Model file for the job. Use its own axes, mm. Coordinates: 2 decimals unless noted, no trailing zeros. Write each loop counter-clockwise with the first axis right and the second up, starting at its lowest first coordinate (ties: lowest second). Pieces come first, ordered by that corner, then holes. Notation, with made-up numbers: M 66.25,-24.75 L 72.25,-24.75 A21 ccw 72.25,-9.75 Z; hole C -34,83 d10. An arc over 180 degrees is marked long. Put each result on its own line as item: value. Start each with the question number.
Q1. Cut at B-B (x = 92.5). Write the cut outline in (y, z).
Q2. Drill centre lines: line 1 along X through (y, z) = (2.9, -72); line 2 along X through (y, z) = (0.85, -36.83); line 3 along Z through (x, y) = (157, 1.9). Where is each one in solid material? Low to high.
Q3. Cut at C-C (z = -146.5). Write the cut outline in (x, y), then the cut area to 3 significant figures.
Q4. Drop flat-ended pins along their axis: pin 1 (4 mm diameter, centred on x = 68.072, z = -52.705, fed in from -Y); pin 2 (1.5 mm diameter, centred on y = 1, z = -170.5, fed in from -X). Give the stop position or say it passes through.
Q5. Cut at A-A (y = 2.6). Give the number of separate pieces and of enclosed holes in the cut face, then the cut area to 3 significant figures.
```python
from build123d import *

# Parameters (mm, degrees)
BOSS_EXTRUDE1_DEPTH   = 3.0734
COMPRESSOR_MOUNTS_D   = 4.4958
F_8_CLEARANCE_HOLE2_D = 4.4958
FILLET1_R             = 3.81
CUT_EXTRUDE1_DEPTH    = 4.0734


with BuildPart() as part:
    # Sketch1 → Boss-Extrude1 (new body)
    with BuildSketch(Plane(origin=(0, 0, 0), x_dir=(1, 0, 0), z_dir=(0, 1, 0))):
        Polygon((0, 0), (281.94, 0), (281.94, 191.77), (224.79, 191.77), (224.79, 128.27), (0, 128.27), align=None)
    extrude(amount=BOSS_EXTRUDE1_DEPTH)

    # Compressor Mounts (through all)
    with Locations(Plane(origin=(0, 3.0734, 0), x_dir=(1, 0, 0), z_dir=(0, 1, 0))):
        with Locations((140.6525, 38.835), (107.743534656, 95.835), (173.561465344, 95.835)):
            Hole(COMPRESSOR_MOUNTS_D / 2)

    # #8 Clearance Hole2 (through all)
    with Locations(Plane(origin=(0, 3.0734, 0), x_dir=(1, 0, 0), z_dir=(0, 1, 0))):
        with Locations((12.7, 11.635), (269.24, 11.635), (269.24, 179.07), (12.7, 116.635), (173.561465344, 64.135), (140.6525, 38.835), (107.743534656, 95.835), (173.561465344, 95.835), (212.344, 20.32), (68.072, 103.505), (68.072, 52.705), (43.18, 36.83), (226.06, 27.432)):
            Hole(F_8_CLEARANCE_HOLE2_D / 2)

    # Fillet1
    fillet1_edges = [part.edges().sort_by_distance(p)[0] for p in [
        (0, 1.5367, -128.27),
        (224.79, 1.5367, -128.27),
        (224.79, 1.5367, -191.77),
        (281.94, 1.5367, -191.77),
        (281.94, 1.5367, 0),
        (0, 1.5367, 0),
    ]]
    fillet(fillet1_edges, radius=FILLET1_R)

    # Sketch7 → Cut-Extrude1 (cut, through all)
    with BuildSketch(Plane(origin=(0, 3.0734, 0), x_dir=(1, 0, 0), z_dir=(0, 1, 0))):
        with BuildLine():
            Line((243.8019, 179.07), (243.8019, 153.67))
            ThreePointArc((243.8019, 153.67), (241.554, 151.4221), (239.3061, 153.67))
            Line((239.3061, 153.67), (239.3061, 179.07))
            ThreePointArc((239.3061, 179.07), (241.554, 181.3179), (243.8019, 179.07))
        make_face()
        with BuildLine():
            Line((243.8019, 48.67), (243.8019, 74.07))
            ThreePointArc((243.8019, 74.07), (241.554, 76.3179), (239.3061, 74.07))
            Line((239.3061, 74.07), (239.3061, 48.67))
            ThreePointArc((239.3061, 48.67), (241.554, 46.4221), (243.8019, 48.67))
        make_face()
    extrude(amount=-CUT_EXTRUDE1_DEPTH, mode=Mode.SUBTRACT)


solid = part.part
```
Computed values:
1. outline: M 0,-128.27 L 3.07,-128.27 L 3.07,0 L 0,0 Z
2. line 1: 0 to 239.31, 243.8 to 281.94
2. line 2: 0 to 40.93, 45.43 to 139.64, 141.67 to 281.94
2. line 3: -128.27 to 0
3. outline: M 224.79,0 L 281.94,0 L 281.94,3.07 L 224.79,3.07 Z
3. area: 176 mm2
4. pin 1: through
4. pin 2: x = 224.79
5. separate pieces: 1
5. enclosed holes: 15
5. area: 39,300 mm2
